Verification items for the finished model (mm, model axes). A direction names the side the tool comes from. Round coordinates to 2 decimals unless told otherwise and drop trailing zeros. Write each loop counter-clockwise with the first axis right and the second up, starting at its lowest first coordinate (ties: lowest second). Pieces come first, ordered by that corner, then holes. Notation, with made-up numbers: (-15.75, -38) -> (-1.75, -38) arc R8 ccw to (-1.75, -25) -> close; hole circle Ø11 at (27, 89). An arc over 180 degrees is marked (long way). Answer as a JSON object with one key per item and string values. Group by question number.
(1) Sectioned sample at D-D on y = 8. Record the cut outline in (x, z), and give its area (3 significant figures).
(2) Draft check along Z on faces 5 (the face through (-6, -21, 25.7)), 6 (the face through (-6, 0, 54)), 7 (the face through (-9, 0, 1)). Enter one of: released by +Z, released by -Z, zero draft, split by the parting line, or undercut.
(3) Gauge pin test, flat ends, axial feed: pin 1 Ø2 at (x, y) = (0, 20) entering from -Z; pin 2 Ø4 at (x, y) = (-1.5, 19.5) entering from +Z; pin 3 Ø4 at (y, z) = (19, 15.5) entering from +X; pin 4 Ø6 at (x, z) = (2.5, 10) entering from -Y. Record the tip position at first contact, or that the pin passes through.
(4) Scan lines: L1, parallel to Y at x = 0, z = 2.45; L2, parallel to X at y = -20, z = 1.85; L3, parallel to Z at x = -5.25, y = 16.5. Record each from-to range of solid material in increasing order. Write a range as from..to.
(5) Sectioned sample at A-A on x = 0. Record the cut outline in (y, z), and give its area (3 significant figures).
(6) Sectioned sample at B-B on y = 20. Record the cut outline in (x, z).
(7) Set-up check for faces 1 (the face through (-8, 0, 3)), 2 (the face through (-4.5, 0, 22)), 3 (the face through (-6, -23.1, 28)), 4 (the face through (-1, 26, 7)): record each of +Z, -Z, +X, -X, +Y, -Y from which the full face is reachable in a straight line by a thin tool's end or side.
(8) Sectioned sample at C-C on z = 34.5. Record the cut outline in (x, y), and give its area (3 significant figures).
```python
from build123d import *

# Parameters (mm, degrees)
SKETCH_1_W                         = 18
SKETCH_1_H                         = 54
FOOT_DEPTH                         = 3
UPRIGHT_START                      = 3
SKETCH_2_W                         = 3
SKETCH_2_H                         = 54
UPRIGHT_DEPTH                      = 51
REAR_COMPONENTS_OPEN_WINDOW_START  = -8
SKETCH_3_W                         = 23
SKETCH_3_H                         = 34
REAR_COMPONENTS_OPEN_WINDOW_DEPTH  = 5
SENSOR_M2_SLOTS_CENTRES42X17_START = -8
SKETCH_4_W                         = 3.6
SKETCH_4_H                         = 4.2
SENSOR_M2_SLOTS_CENTRES42X17_DEPTH = 5
SIDE_GUSSET_START                  = -26
SIDE_GUSSET_DEPTH                  = 2
EXTRUDE_START                      = 24
EXTRUDE_4_DEPTH                    = 2
FOOT_M3_HOLES_PITCH40_START        = -0.1
SKETCH_7_R                         = 1.7
FOOT_M3_HOLES_PITCH40_DEPTH        = 3.2


with BuildPart() as part:
    # 草图1 → Foot (new body)
    with BuildSketch(Plane.XY):
        Rectangle(SKETCH_1_W, SKETCH_1_H)
    extrude(amount=FOOT_DEPTH)

    # 草图2 → Upright (add)
    with BuildSketch(Plane.XY.offset(UPRIGHT_START)):
        with Locations((-6, 0)):
            Rectangle(SKETCH_2_W, SKETCH_2_H)
    extrude(amount=UPRIGHT_DEPTH)

    # 草图3 → Rear_components_open_window (cut)
    with BuildSketch(Plane(origin=(0, 0, 0), x_dir=(0, 0, -1), z_dir=(1, 0, 0)).offset(REAR_COMPONENTS_OPEN_WINDOW_START)):
        with Locations((-36, 0)):
            Rectangle(SKETCH_3_W, SKETCH_3_H)
    extrude(amount=REAR_COMPONENTS_OPEN_WINDOW_DEPTH, mode=Mode.SUBTRACT)

    # 草图4 → Sensor_M2_slots_centres42x17 (cut)
    with BuildSketch(Plane(origin=(0, 0, 0), x_dir=(0, 0, -1), z_dir=(1, 0, 0)).offset(SENSOR_M2_SLOTS_CENTRES42X17_START)):
        with Locations((-27.5, -21)):
            Rectangle(SKETCH_4_W, SKETCH_4_H)
        with Locations((-44.5, -21)):
            Rectangle(SKETCH_4_W, SKETCH_4_H)
        with Locations((-27.5, 21)):
            Rectangle(SKETCH_4_W, SKETCH_4_H)
        with Locations((-44.5, 21)):
            Rectangle(SKETCH_4_W, SKETCH_4_H)
    extrude(amount=SENSOR_M2_SLOTS_CENTRES42X17_DEPTH, mode=Mode.SUBTRACT)

    # 草图5 → Side_gusset (add)
    with BuildSketch(Plane(origin=(0, 0, 0), x_dir=(1, 0, 0), z_dir=(0, 1, 0)).offset(SIDE_GUSSET_START)):
        Polygon((-4.5, -3), (8, -3), (-4.5, -16), align=None)
    extrude(amount=SIDE_GUSSET_DEPTH)

    # 草图6 → 凸台-拉伸4 (add)
    with BuildSketch(Plane(origin=(0, 0, 0), x_dir=(1, 0, 0), z_dir=(0, 1, 0)).offset(EXTRUDE_START)):
        Polygon((-4.5, -3), (8, -3), (-4.5, -16), align=None)
    extrude(amount=EXTRUDE_4_DEPTH)

    # 草图7 → Foot_M3_holes_pitch40 (cut)
    with BuildSketch(Plane.XY.offset(FOOT_M3_HOLES_PITCH40_START)):
        with Locations((0, -20)):
            Circle(SKETCH_7_R)
        with Locations((0, 20)):
            Circle(SKETCH_7_R)
    extrude(amount=FOOT_M3_HOLES_PITCH40_DEPTH, mode=Mode.SUBTRACT)


solid = part.part
```
Computed values:
{
 "1": {"outline": "(-9, 0) -> (9, 0) -> (9, 3) -> (-4.5, 3) -> (-4.5, 24.5) -> (-7.5, 24.5) -> (-7.5, 3) -> (-9, 3) -> close; (-7.5, 47.5) -> (-4.5, 47.5) -> (-4.5, 54) -> (-7.5, 54) -> close", "area": "138 mm2"},
 "2": {"face 5": "undercut", "face 6": "released by +Z", "face 7": "zero draft"},
 "3": {"pin 1": "through", "pin 2": "z = 3", "pin 3": "x = -4.5", "pin 4": "y = -26"},
 "4": {"L1": "-27..-21.7, -18.3..18.3, 21.7..27", "L2": "-9..-1.7, 1.7..9", "L3": "0..24.5, 47.5..54"},
 "5": {"outline": "(-27, 0) -> (-21.7, 0) -> (-21.7, 3) -> (-24, 3) -> (-24, 11.32) -> (-26, 11.32) -> (-26, 3) -> (-27, 3) -> close; (-18.3, 0) -> (18.3, 0) -> (18.3, 3) -> (-18.3, 3) -> close; (21.7, 0) -> (27, 0) -> (27, 3) -> (26, 3) -> (26, 11.32) -> (24, 11.32) -> (24, 3) -> (21.7, 3) -> close", "area": "175 mm2"},
 "6": {"outline": "(-9, 0) -> (-1.7, 0) -> (-1.7, 3) -> (-4.5, 3) -> (-4.5, 25.7) -> (-7.5, 25.7) -> (-7.5, 3) -> (-9, 3) -> close; (-7.5, 29.3) -> (-4.5, 29.3) -> (-4.5, 42.7) -> (-7.5, 42.7) -> close; (-7.5, 46.3) -> (-4.5, 46.3) -> (-4.5, 54) -> (-7.5, 54) -> close; (1.7, 0) -> (9, 0) -> (9, 3) -> (1.7, 3) -> close"},
 "7": {"face 1": "+Z, -X, +Y, -Y", "face 2": "+Z, +X", "face 3": "+X, -X", "face 4": "+Z, +X, +Y"},
 "8": {"outline": "(-7.5, -27) -> (-4.5, -27) -> (-4.5, -17) -> (-7.5, -17) -> close; (-7.5, 17) -> (-4.5, 17) -> (-4.5, 27) -> (-7.5, 27) -> close", "area": "60.0 mm2"}
}
